Autodesk Inventor part; units mm, degrees
ref_plane "YZ Plane" through (0, 0, 0) normal (1, 0, 0) x (0, 1, 0)
ref_plane "XZ Plane" through (0, 0, 0) normal (0, 1, 0) x (-1, 0, 0)
ref_plane "XY Plane" through (0, 0, 0) normal (0, 0, 1) x (1, 0, 0)
sketch "Sketch1" plane through (0, 0, 0) normal (0, 1, 0) x (-1, 0, 0)
  line L0 (0, 0) -> (-14.5, 0)
  line L1 (-14.5, 0) -> (-14.5, -42.5)
  line L2 (-14.5, -42.5) -> (0, -42.5)
  line L3 (0, -42.5) -> (0, 0)
  line L4 (0, 0) -> (15.5, 0)
  line L5 (15.5, 0) -> (15.5, -17.25)
  line L6 (15.5, -17.25) -> (0, -17.25)
  line L7 (0, -17.25) -> (0, 0)
  line L8 (0, -17.25) -> (10, -17.25)
  line L9 (10, -17.25) -> (10, -18.25)
  line L10 (10, -18.25) -> (0, -18.25)
  line L11 (0, -18.25) -> (0, -17.25)
  line L12 (0, -17.25) -> (1, -17.25)
  line L13 (1, -17.25) -> (1, -27.25)
  line L14 (1, -27.25) -> (0, -27.25)
  line L15 (0, -27.25) -> (0, -17.25)
  line L16 (10, 0) -> (-14.5, 0)
  line L17 (-14.5, 0) -> (-14.5, 1)
  line L18 (-14.5, 1) -> (10, 1)
  line L19 (10, 1) -> (10, 0)
  line L20 (-14.5, 1) -> (-15.5, 1)
  line L21 (-15.5, 1) -> (-15.5, -27.25)
  line L22 (-15.5, -27.25) -> (-14.5, -27.25)
  line L23 (-14.5, -27.25) -> (-14.5, 1)
  line L24 (11.7177, -28.7701) -> (-19.9895, -28.7701)
  line L25 (-19.9895, -28.7701) -> (-19.9895, 4.2767)
  line L26 (-19.9895, 4.2767) -> (11.7177, 4.2767)
  line L27 (11.7177, 4.2767) -> (11.7177, -28.7701)
  dimension "d0" = 15.5
  dimension "d1" = 17.25
  dimension "d2" = 14.5
  dimension "d3" = 42.5
  dimension "d4" = 1
  dimension "d5" = 10
  dimension "d6" = 10
  dimension "d7" = 1
  dimension "d8" = 1
  dimension "d9" = 1
  dimension "d10" = 28.25
extrude "Extrusion1" add sketch "Sketch1" against normal blind 1 contours L3 L24 L1 L0 | L4 L27 L6 L3 | L0 L17 L18 L19 L4 | L1 L22 L21 L20 L17 | L6 L13 L10 L3 | L19 L18 L20 L21 L22 L1 L24 L25 L26 L27 L4 | L10 L13 L14 L3 | L6 L9 L10 L13 | L14 L13 L10 L9 L6 L27 L24 L3
extrude "Extrusion2" add sketch "Sketch1" along normal blind 7 contours L0 L17 L18 L19 L4 | L1 L22 L21 L20 L17 | L6 L13 L10 L3 | L10 L13 L14 L3 | L6 L9 L10 L13
sketch "Sketch2" plane through (-10, 0, -17.25) normal (-1, 0, 0) x (0, 0, 1)
  line L0 (0, 0) -> (-1, 0)
  line L1 (0, 0) -> (0, 7)
  line L2 (-1, 7) -> (0, 7)
  line L3 (-1, 0) -> (-1, 7)
  line L4 (18.25, 0) -> (17.25, 0)
  line L5 (18.25, 0) -> (18.25, 7)
  line L6 (17.25, 7) -> (18.25, 7)
  line L7 (17.25, 0) -> (17.25, 7)
  arc A0 (0, 4.027) -> (17.25, 4.027) centre (8.625, 11.25) ccw
  line L8 (21.5267, 0) -> (-11.5201, 0)
  line L9 (17.25, 4.027) -> (17.25, 0)
  line L10 (17.25, 0) -> (0, 0)
  line L11 (0, 0) -> (0, 4.027)
  line L12 (0, 0) -> (0, 7)
  line L13 (0, 4.027) -> (0, 0)
  line L14 (0, 0) -> (17.25, 0)
  line L15 (17.25, 0) -> (17.25, 4.027)
  arc A1 (0, 4.027) -> (17.25, 4.027) centre (8.625, 11.25) ccw
  line L16 (17.25, 4.027) -> (17.25, 0)
  line L17 (17.25, 0) -> (0, 0)
  line L18 (0, 0) -> (0, 4.027)
  line L19 (0, 4.027) -> (0, 0)
  line L20 (0, 0) -> (8.625, 0)
  line L21 (8.625, 0) -> (17.25, 0)
  line L22 (-11.5201, 0) -> (21.5267, 0)
  line L23 (17.25, 0) -> (17.25, 4.027)
  dimension "d15" = 8.625
  dimension "d16" = 22.5
sketch "Sketch3" plane through (-10, 0, -17.25) normal (-1, 0, 0) x (0, 0, 1)
  line L0 (0, 0) -> (-1, 0)
  line L1 (0, 0) -> (0, 7)
  line L2 (-1, 7) -> (0, 7)
  line L3 (-1, 0) -> (-1, 7)
  line L4 (18.25, 0) -> (17.25, 0)
  line L5 (18.25, 0) -> (18.25, 7)
  line L6 (17.25, 7) -> (18.25, 7)
  line L7 (17.25, 0) -> (17.25, 7)
  line L8 (21.5267, 0) -> (-11.5201, 0)
  arc A0 (0, 4.1686) -> (17.25, 4.1686) centre (8.625, 11.007) ccw
  line L9 (-11.5201, 0) -> (21.5267, 0)
  line L10 (0, 0) -> (0, 7)
  line L11 (0, 4.1686) -> (0, 0)
  line L12 (0, 0) -> (8.625, 0)
  line L13 (18.25, 0) -> (17.25, 0)
  line L14 (8.625, 0) -> (17.25, 0)
  line L15 (17.25, 0) -> (17.25, 4.1686)
  dimension "d17" = 8.625
extrude "Extrusion3" add sketch "Sketch3" against normal blind 10 contours A0 L7 L8 | L1 A0 L8
properties part number "motor_mount_fitcheck1"
The model under review builds one solid part; all positions refer to its coordinate system, in mm. A direction names the side the tool comes from. Round coordinates to 2 decimals unless told otherwise and drop trailing zeros. Order: outer loops, then holes, each group sorted by start corner. A loop starts at its lowest first (then second) coordinate and runs counter-clockwise, first axis right, second up. Notation, with made-up numbers: (-2, 89) -> (45, 89) arc R12 cw to (45, 97) -> close; hole circle Ø7 at (-21, 43.25). An arc over 180 degrees is marked (long way). One line per item, written item: value. Start each with the question number.
Q1. Take a section at A-A (y = 6.5). Write out the cut boundary in (x, z), and give its area (4 significant figures).
Q2. Mouldability with a two-part tool opening along Z and no side actions: class faces 6 (the face through (3.9, -0.5, -28.77)), 7 (the face through (-5, 6, -17.25)), 8 (the face through (0, 4, -22)) as released by +Z, released by -Z, zero draft, split by the parting line, or undercut.
Q3. Wall thickness on line 1 (X direction, y = 6.75, z = -19); line 2 (X direction, y = 2.25, z = -1); line 3 (Y direction, x = 1, z = -21.5): over which ranges is each line inside the solid? List them lowest first.
Q4. Machinability: for faces 1 (the face through (-6, 3, -18.25)), 2 (the face through (-5.1, 0, -8.8)), 3 (the face through (15.5, 3, -13)), 4 (the face through (-0.5, 3.5, -27.25)), 5 (the face through (-10, 2, -16)), which of the approach directions +Z, -Z, +X, -X, +Y, -Y give a long, thin tool a straight path to every point of the face, cutting with its end or side? Answer none if there is none.
Q5. Take a section at C-C (z = -23.5). Write out the cut boundary in (x, y), and give its area (3 significant figures).
Q6. Take a section at B-B (x = -3.5). Write out the cut boundary in (y, z) (3 decimals), and give its area (3 significant figures).
Q7. Clearance check with flat-ended pins moving along their axes: pin 1 Ø2 at (y, z) = (3.5, -13.5) entering from -X; pin 2 Ø2 at (y, z) = (5, -18) entering from +X; pin 3 Ø1.5 at (x, z) = (8, -8.5) entering from +Y; pin 4 Ø10 at (x, z) = (17, 0) entering from +Y. State where each tip first meets the part, or that it passes through.
Q8. Take a section at D-D (x = 2.5). Write out the cut boundary in (y, z), and give its area (3 significant figures).
Reported:
1. outline: (-10, -18.25) -> (-1, -18.25) -> (-1, -27.25) -> (0, -27.25) -> (0, -17.25) -> (-10, -17.25) -> close; (-10, 0) -> (14.5, 0) -> (14.5, -27.25) -> (15.5, -27.25) -> (15.5, 1) -> (-10, 1) -> close
1. area: 71.75 mm2
2. face 6: released by -Z
2. face 7: undercut
2. face 8: zero draft
3. line 1: x = -1 to 0, 14.5 to 15.5
3. line 2: x = -10 to 0, 14.5 to 15.5
3. line 3: y = -1 to 0
4. face 1: -Z, -X, +Y
4. face 2: -X, +Y
4. face 3: +Z, -Z, +X, +Y
4. face 4: -Z, +X, -X, +Y
4. face 5: +Z, -Z, -X, +Y
5. outline: (-11.72, -1) -> (19.99, -1) -> (19.99, 0) -> (15.5, 0) -> (15.5, 7) -> (14.5, 7) -> (14.5, 0) -> (0, 0) -> (0, 7) -> (-1, 7) -> (-1, 0) -> (-11.72, 0) -> close
5. area: 45.7 mm2
6. outline: (-1, -28.77) -> (0, -28.77) -> (0, -18.25) -> (7, -18.25) -> (7, -17.25) -> (4.169, -17.25) arc R11.007 cw to (4.169, 0) -> (7, 0) -> (7, 1) -> (0, 1) -> (0, 4.277) -> (-1, 4.277) -> close
6. area: 68.8 mm2
7. pin 1: stops at x = 14.5
7. pin 2: stops at x = 15.5
7. pin 3: stops at y = 0
7. pin 4: stops at y = 7
8. outline: (-1, -28.77) -> (0, -28.77) -> (0, 0) -> (7, 0) -> (7, 1) -> (0, 1) -> (0, 4.28) -> (-1, 4.28) -> close
8. area: 40.0 mm2
